Design review of the part built by this model. Coordinates are the model's own, in mm. A direction names the side the tool comes from. Round coordinates to 2 decimals unless told otherwise and drop trailing zeros. Loops run counter-clockwise (first coordinate to the right, second up) from the corner with the lowest first, then second, coordinate; pieces in that order, holes last. Notation, with made-up numbers: M 70.25,66.25 L 98.25,66.25 A9 cw 98.25,80.25 Z; hole C -34.75,45.25 d4. An arc over 180 degrees is marked long. One line per item, written item: value. Start each with the question number.
Item 1: Clearance check with flat-ended pins moving along their axes: pin 1 (10 mm diameter, centred on x = 0, y = 7.72, fed in from -Z); pin 2 (3 mm diameter, centred on y = 27.5, z = 18.5, fed in from +X); pin 3 (8 mm diameter, centred on x = -3.5, z = -5, fed in from +Y). State where each tip first meets the part, or that it passes through.
Item 2: We need section C-C (z = 27). Write out the cut boundary in (x, y), then the cut area to 3 significant figures.
Item 3: For faces 1 (the flat face through (18, -28.53, 18)), 2 (the cylindrical face through (-0.7, 4.7, 14.8)), 3 (the flat face through (18, -31, 0)), 4 (the flat face through (-3, -28.53, -4)), list the 3-axis set-ups (+Z, -Z, +X, -X, +Y, -Y) from which the entire face can be reached by the end or side of a thin tool; tool diameter is ignored.
Item 4: We need section B-B (x = 18). Write out the cut boundary in (y, z), then the cut area to 3 significant figures.
Item 5: We need section A-A (z = -7). Write out the cut boundary in (x, y), then the cut area to 3 significant figures.
Item 6: Mouldability with a two-part tool opening along Z and no side actions: class faces 5 (the flat face through (0, 11, 0)), 6 (the cylindrical face through (20.957, -31.065, 8.931)), 7 (the cylindrical face through (-0.404, 38.793, 14.79)) as released by +Z, released by -Z, zero draft, split by the parting line, or undercut.
Item 7: For line 1 along Z through (x, y) = (18, -31.6); line 2 along Y through (x, z) = (0, 8.5); line 3 along X through (y, z) = (8, 5), list the stretches that pass through material, from the lowest coordinate up.
Item 8: We need section D-D (x = 0). Write out the cut boundary in (y, z), then the cut area to 3 significant figures.
from build123d import *

# Parameters (mm, degrees)
SKETCH1_W           = 22
SKETCH1_H           = 82.75
SKETCH1_R           = 3.1
BOSS_EXTRUDE1_DEPTH = 30
SKETCH2_W           = 22
SKETCH2_H           = 82.75
BOSS_EXTRUDE2_DEPTH = 5
SKETCH3_W           = 22
SKETCH3_H           = 14
SKETCH3_R           = 3.1
SKETCH3_W_2         = 14
SKETCH3_H_2         = 35
BOSS_EXTRUDE3_DEPTH = 5


with BuildPart() as part:
    # Sketch1 → Boss-Extrude1 (new body)
    with BuildSketch(Plane.XY):
        with Locations((0, 7.844654309)):
            Rectangle(SKETCH1_W, SKETCH1_H)
        with Locations((0, 35.719654309)):
            Circle(SKETCH1_R, mode=Mode.SUBTRACT)
        with Locations((0, 7.719654309)):
            Circle(SKETCH1_R, mode=Mode.SUBTRACT)
    extrude(amount=BOSS_EXTRUDE1_DEPTH)

    # Sketch2 → Boss-Extrude2 (add)
    with BuildSketch(Plane.XY.offset(30)):
        with Locations((0, 7.844654309)):
            Rectangle(SKETCH2_W, SKETCH2_H)
    extrude(amount=BOSS_EXTRUDE2_DEPTH)

    # Sketch3 → Boss-Extrude3 (add)
    with BuildSketch(Plane.XZ.offset(33.530345691)):
        with Locations((0, -7)):
            Rectangle(SKETCH3_W, SKETCH3_H)
        with Locations((0, -7)):
            Circle(SKETCH3_R, mode=Mode.SUBTRACT)
        with Locations((18, 17.5)):
            Rectangle(SKETCH3_W_2, SKETCH3_H_2)
        with Locations((18, 27)):
            Circle(SKETCH3_R, mode=Mode.SUBTRACT)
        with Locations((18, 8)):
            Circle(SKETCH3_R, mode=Mode.SUBTRACT)
    extrude(amount=-BOSS_EXTRUDE3_DEPTH)


solid = part.part
A:
1. pin 1: z = 0
1. pin 2: x = 11
1. pin 3: y = -28.53
2. outline: M -11,-33.53 L 14.9,-33.53 L 14.9,-28.53 L 11,-28.53 L 11,49.22 L -11,49.22 Z; M 21.1,-33.53 L 25,-33.53 L 25,-28.53 L 21.1,-28.53 Z; hole C 0,7.72 d6.2; hole C 0,35.72 d6.2
2. area: 1,800 mm2
3. face 1: +Z, -Z, +X, +Y
3. face 2: -Z
3. face 3: -Z, +X, +Y, -Y
3. face 4: -Z, +X, -X, +Y
4. outline: M -33.53,0 L -28.53,0 L -28.53,4.9 L -33.53,4.9 Z; M -33.53,11.1 L -28.53,11.1 L -28.53,23.9 L -33.53,23.9 Z; M -33.53,30.1 L -28.53,30.1 L -28.53,35 L -33.53,35 Z
4. area: 113 mm2
5. outline: M -11,-33.53 L -3.1,-33.53 L -3.1,-28.53 L -11,-28.53 Z; M 3.1,-33.53 L 11,-33.53 L 11,-28.53 L 3.1,-28.53 Z
5. area: 79.0 mm2
6. face 5: released by -Z
6. face 6: undercut
6. face 7: zero draft
7. line 1: 0 to 4.9, 11.1 to 23.9, 30.1 to 35
7. line 2: -33.53 to 4.62, 10.82 to 32.62, 38.82 to 49.22
7. line 3: -11 to -3.09, 3.09 to 11
8. outline: M -33.53,-14 L -28.53,-14 L -28.53,-10.1 L -33.53,-10.1 Z; M -33.53,-3.9 L -28.53,-3.9 L -28.53,0 L 4.62,0 L 4.62,30 L 10.82,30 L 10.82,0 L 32.62,0 L 32.62,30 L 38.82,30 L 38.82,0 L 49.22,0 L 49.22,35 L -33.53,35 Z
8. area: 2,560 mm2
